Part model, mm, in its own coordinate system. Give positions to 0.01 mm unless a question says otherwise; leave off trailing zeros. Order: outer loops, then holes, each group sorted by start corner. A loop starts at its lowest first (then second) coordinate and runs counter-clockwise, first axis right, second up. Notation, with made-up numbers: M 88,-26.5 L 132,-26.5 A18 ccw 132,-6.5 Z; hole C 5,26 d11. An arc over 180 degrees is marked long. Return JSON: item names as keys, results as strings.
from build123d import *

# Parameters (mm, degrees)
F3_DEPTH = 233.68
F4_DEPTH = 241.3


with BuildPart() as f1:
    # F0 (on Front) → F1 (revolve)
    with BuildSketch(Plane.XZ):
        with BuildLine():
            Line((0, 131.807907), (0, -131.807907))
            ThreePointArc((0, -131.807907), (131.807907, 0), (0, 131.807907))
        make_face()
    revolve(axis=Axis((0, 0, 0), (0, 0, 1)))

    # F2 (on Front) → F3 (cut)
    with BuildSketch(Plane.XZ):
        with BuildLine():
            Line((-127.972643, 14.135387), (0, 0))
            Line((0, 0), (-103.759866, 76.227926))
            ThreePointArc((-103.759866, 76.227926), (-119.953573, 46.775493), (-127.972643, 14.135387))
        make_face()
        with BuildLine():
            Line((-117.895253, -51.744717), (0, 0))
            Line((0, 0), (-127.972643, 14.135387))
            ThreePointArc((-127.972643, 14.135387), (-127.270588, -19.468022), (-117.895253, -51.744717))
        make_face()
    extrude(amount=-F3_DEPTH, mode=Mode.SUBTRACT)

    # F2 (on Front) → F4 (cut)
    with BuildSketch(Plane.XZ):
        with BuildLine():
            Line((-127.972643, 14.135387), (0, 0))
            Line((0, 0), (-103.759866, 76.227926))
            ThreePointArc((-103.759866, 76.227926), (-119.953573, 46.775493), (-127.972643, 14.135387))
        make_face()
        with BuildLine():
            Line((-117.895253, -51.744717), (0, 0))
            Line((0, 0), (-127.972643, 14.135387))
            ThreePointArc((-127.972643, 14.135387), (-127.270588, -19.468022), (-117.895253, -51.744717))
        make_face()
    extrude(amount=F4_DEPTH, mode=Mode.SUBTRACT)


solid = f1.part
Q1. Band-saw the part on D-D (x = 6). Give the cut face in (y, z).
Established:
{"outline": "C 0,0 d263.34"}
Q2. Pin check, flat tips, straight feed: pin 1 (8 mm diameter, centred on x = -29, y = 83.5, fed in from -Z); pin 2 (4 mm diameter, centred on y = 103.5, z = -37, fed in from +X); pin 3 (1.5 mm diameter, centred on x = 35.5, z = 71, fed in from -Y). Stop position of each tip, or through.
Established:
{"pin 1": "stops at z = -101.25", "pin 2": "stops at x = 75.68", "pin 3": "stops at y = -105.79"}
Q3. Band-saw the part on C-C (y = -83.5). Give the cut face in (x, z).
Established:
{"outline": "M -93.39,-40.99 A101.99 ccw long -82.19,60.38 L 0,0 Z"}
Q4. Band-saw the part on A-A (z = 44). Give the cut face in (x, y), then the cut area to 3 significant figures.
Established:
{"outline": "M -121,-28.22 L -121,28.22 A124.25 ccw Z; M -59.89,-108.86 A124.25 ccw long -59.89,108.86 Z", "area": "38,700 mm²"}
Q5. Band-saw the part on B-B (x = -24.5). Give the cut face in (y, z).
Established:
{"outline": "M -129.06,-10.75 A129.51 ccw 129.06,-10.75 Z; M -128.25,18 L 128.25,18 A129.51 ccw Z"}
Q6. Probe line 1 along Z through (x, y) = (-88.5, -65.5); line 2 along Z through (x, y) = (-84.5, -6); line 3 along X through (y, z) = (-120, 9.5). List the from-to ranges inside material, lowest first.
Established:
{"line 1": "z = -72.46 to -38.84, 65.02 to 72.46", "line 2": "z = -100.98 to -37.09, 62.08 to 100.98", "line 3": "x = -12.93 to 53.69"}
